Verification items for the finished model (mm, model axes). Round coordinates to 2 decimals unless told otherwise and drop trailing zeros. Loops run counter-clockwise (first coordinate to the right, second up) from the corner with the lowest first, then second, coordinate; pieces in that order, holes last. Notation, with made-up numbers: M 88.25,15.25 L 99.25,15.25 A23 ccw 99.25,52.25 Z; hole C 49,61 d4. An arc over 180 degrees is marked long. One line per item, written item: value.
from build123d import *

# Parameters (mm, degrees)
SKETCH1_R           = 1.6
SKETCH1_R_2         = 4
BOSS_EXTRUDE1_DEPTH = 1


with BuildPart() as part:
    # Sketch1 → Boss-Extrude1 (new body, symmetric)
    with BuildSketch(Plane.XY):
        Polygon((-58.447822699, 2.25215401), (205.719516193, 2.25215401), (261.946581062, 26.347260557), (271.703456729, 162.25215401), (-78.296543271, 162.25215401), align=None)
        with Locations((169.158925411, 40.547600357)):
            Circle(SKETCH1_R, mode=Mode.SUBTRACT)
        with Locations((169.158925411, 52.547600357)):
            Circle(SKETCH1_R, mode=Mode.SUBTRACT)
        with Locations((220.457146693, 46.547600357)):
            Circle(SKETCH1_R, mode=Mode.SUBTRACT)
        with Locations((-65.674373942, 150.94432728)):
            Circle(SKETCH1_R_2, mode=Mode.SUBTRACT)
        with Locations((253.311068017, 150.94432728)):
            Circle(SKETCH1_R_2, mode=Mode.SUBTRACT)
        with Locations((251.787322425, 34.458331013)):
            Circle(SKETCH1_R_2, mode=Mode.SUBTRACT)
        with Locations((202.012846736, 15.25215401)):
            Circle(SKETCH1_R_2, mode=Mode.SUBTRACT)
        with Locations((-49.126516792, 10.545043982)):
            Circle(SKETCH1_R_2, mode=Mode.SUBTRACT)
    extrude(amount=BOSS_EXTRUDE1_DEPTH, both=True)


solid = part.part
(1) Sectioned sample at C-C on y = 71.5. Enter the section's corners in (x, z), and give its area (3 significant figures).
Completed:
outline: M -67.04,-1 L 265.19,-1 L 265.19,1 L -67.04,1 Z
area: 664 mm^2
(2) Mould release check, pull along X, two halves, no side actions. Record for faces 1 (the face through (-66.2, 154.91, -0.01)), 2 (the face through (-68.51, 83.37, 0.01)), 3 (the face through (266.757, 93.348, 0.014)): +X half, -X half, draft (parallel to the pull), parting line (faces both ways), or undercut.
Completed:
face 1: undercut
face 2: -X half
face 3: +X half
(3) Thickness scan on L1, parallel to X at y = 37.5, z = -0.05; L2, parallel to Y at x = -48, z = -0.8; L3, parallel to Y at x = -50.5, z = 0. Record the ranges inside material, lowest first. Write a range as from..to.
Completed:
L1: x = -62.82..249.19, 254.39..262.75
L2: y = 2.25..6.71, 14.38..162.25
L3: y = 2.25..6.79, 14.3..162.25
(4) Sectioned sample at A-A on z = 0.4. Count the separate pieces of the cut face and the enclosed holes in it, and give its area (3 significant figures).
Completed:
separate pieces: 1
enclosed holes: 8
area: 52,600 mm^2
(5) Depth check by flat-ended pin: pin 1 Ø2.5 at (x, y) = (169.16, 52.55) entering from +Z. Enter the tip coordinate at first touch or a pass-through.
Completed:
pin 1: passes through
(6) Sectioned sample at B-B on x = 228. Enter the section's corners in (y, z), and give its area (3 significant figures).
Completed:
outline: M 11.8,-1 L 162.25,-1 L 162.25,1 L 11.8,1 Z
area: 301 mm^2
